Could you check a few things on this model? Use its own coordinates, in mm. Face numbers are marked on the shaded views. A direction names the side the tool comes from. Give positions to 0.01 mm unless a question says otherwise; leave off trailing zeros. Loops run counter-clockwise (first coordinate to the right, second up) from the corner with the lowest first, then second, coordinate; pieces in that order, holes last. Notation, with made-up numbers: M 63.25,-35.75 L 121.25,-35.75 A16 ccw 121.25,-13.75 Z; hole C 37.5,70 d1. An arc over 180 degrees is marked long. Answer in a Markdown table with one row per item. Add a question column.
1. I need wall thicknesses on line 1 along X through (y, z) = (-2.5, 13); line 2 along X through (y, z) = (-17.5, 19); line 3 along Z through (x, y) = (-15, -4.5). Which ranges of each line are inside material? Lowest first, please. Write a range as from..to.
2. Which directions (+Z, -Z, +X, -X, +Y, -Y) give clear straight access to the entire face, cutting with the end or side of a thin tool? Please do the marked faces 5 and 6.
3. I'm going to push flat-ended pins straight in: pin 1 Ø3.5 at (y, z) = (-38, 16) entering from +X; pin 2 Ø5 at (y, z) = (-13, 3) entering from +X; pin 3 Ø0.9 at (y, z) = (-38, 8.5) entering from +X. Where does each tip first touch, or does it pass through?
4. If we section it at C-C on z = 7.25: List the corners of the cut face in (x, y) for me.
5. If we section it at A-A on z = 11.25: List the corners of the cut face in (x, y) for me, then the cut area to 3 significant figures.
6. Thinking about a two-plate mould opening in Z: for the marked faces 1, 2, 3 and 4, which applies, released by +Z, released by -Z, zero draft, split by the parting line, or undercut?
7. If we section it at B-B on x = -8: List the corners of the cut face in (y, z) for me.
8. If we section it at D-D on x = 2: List the corners of the cut face in (y, z) for me.
```python
from build123d import *

# Parameters (mm, degrees)
F0_W          = 54.9165850133
F0_H          = 29.332328558
F1_DEPTH      = 25
F2_W          = 54.8067912459
F2_H          = 9.8693305627
F3_DEPTH      = 10
F3_DEPTH_BACK = 25
F4_DEPTH      = 3
F5_R          = 5
F6_W          = 44.9165850133
F6_H          = 6.1664939672
F6_H_2        = 4.8576648161
F7_DEPTH      = 3


with BuildPart() as f1:
    # F0 (on Top) → F1 (new body)
    with BuildSketch(Plane.XY):
        with Locations((-0.0417074934, -24.666164279)):
            Rectangle(F0_W, F0_H)
        Polygon((27.5, 10), (-27.5, 10), (-27.5, -10), (27.4165850133, -10), (27.5, -10), align=None)
        Polygon((-22.7641869603, -1.5628831632), (-22.7355900026, 1.6124145468), (-19.9714030424, 3.17529771), (-17.2358130397, 1.5628831632), (-17.2644099974, -1.6124145468), (-20.0285969576, -3.17529771), align=None, mode=Mode.SUBTRACT)
        Polygon((2.7641869603, 1.5628831632), (2.7355900026, -1.6124145468), (-0.0285969576, -3.17529771), (-2.7641869603, -1.5628831632), (-2.7355900026, 1.6124145468), (0.0285969576, 3.17529771), align=None, mode=Mode.SUBTRACT)
        Polygon((22.7641869603, 1.5628831632), (22.7355900026, -1.6124145468), (19.9714030424, -3.17529771), (17.2358130397, -1.5628831632), (17.2644099974, 1.6124145468), (20.0285969576, 3.17529771), align=None, mode=Mode.SUBTRACT)
    extrude(amount=F1_DEPTH)

    # F2 (on Front) → F3 (cut, two sides)
    with BuildSketch(Plane.XZ) as f3_sk:
        with Locations((-0.1290403306, 4.9346652813)):
            Rectangle(F2_W, F2_H)
    extrude(amount=F3_DEPTH, mode=Mode.SUBTRACT)
    extrude(f3_sk.sketch, amount=-F3_DEPTH_BACK, mode=Mode.SUBTRACT)

    # F0 (on Top) → F4 (join)
    with BuildSketch(Plane.XY):
        Polygon((27.5, 10), (-27.5, 10), (-27.5, -10), (27.4165850133, -10), (27.5, -10), align=None)
        Polygon((-22.7641869603, -1.5628831632), (-22.7355900026, 1.6124145468), (-19.9714030424, 3.17529771), (-17.2358130397, 1.5628831632), (-17.2644099974, -1.6124145468), (-20.0285969576, -3.17529771), align=None, mode=Mode.SUBTRACT)
        Polygon((2.7641869603, 1.5628831632), (2.7355900026, -1.6124145468), (-0.0285969576, -3.17529771), (-2.7641869603, -1.5628831632), (-2.7355900026, 1.6124145468), (0.0285969576, 3.17529771), align=None, mode=Mode.SUBTRACT)
        Polygon((22.7641869603, 1.5628831632), (22.7355900026, -1.6124145468), (19.9714030424, -3.17529771), (17.2358130397, -1.5628831632), (17.2644099974, 1.6124145468), (20.0285969576, 3.17529771), align=None, mode=Mode.SUBTRACT)
    extrude(amount=F4_DEPTH)

    # F5
    f5_edges = [f1.edges().sort_by_distance(p)[0] for p in [
        (-0.041707, -39.332329, 25),
        (-0.041707, -39.332329, 0),
        (27.416585, -39.332329, 12.5),
        (-27.5, -39.332329, 12.5),
    ]]
    fillet(f5_edges, radius=F5_R)

    # F6 (on face) → F7 (cut)
    with BuildSketch(Plane.XZ.offset(39.332328558)):
        with Locations((-0.0417074934, 16.9167530164)):
            Rectangle(F6_W, F6_H)
        with Locations((-0.0417074934, 7.428832408)):
            Rectangle(F6_W, F6_H_2)
    extrude(amount=-F7_DEPTH, mode=Mode.SUBTRACT)


solid = f1.part
```
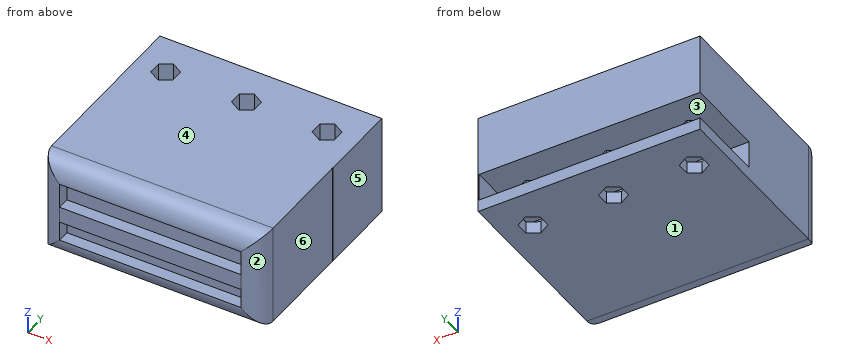
Results:
| question | item | result |
|---|---|---|
| 1 | line 1 | -27.5..-21.17, -18.83..-1.17, 1.17..18.83, 21.17..27.5 |
| 1 | line 2 | -27.5..27.42 |
| 1 | line 3 | 0..3, 9.87..25 |
| 2 | face 5 | +Z, -Z, +X, +Y, -Y |
| 2 | face 6 | +Z, -Z, +X, -Y |
| 3 | pin 1 | x = 27.03 |
| 3 | pin 2 | x = 27.42 |
| 3 | pin 3 | x = 26.24 |
| 4 | outline | M -27.5,-34.33 A5 ccw -22.5,-39.33 L -22.5,-36.33 L 22.42,-36.33 L 22.42,-39.33 A5 ccw 27.42,-34.33 L 27.42,-10 L 27.5,-10 L 27.5,10 L 27.27,10 L 27.27,-10 L -27.5,-10 Z |
| 5 | outline | M -27.5,-34.33 A5 ccw -22.5,-39.33 L 22.42,-39.33 A5 ccw 27.42,-34.33 L 27.42,-10 L 27.5,-10 L 27.5,10 L -27.5,10 Z; hole M -22.76,-1.56 L -20.03,-3.18 L -17.26,-1.61 L -17.24,1.56 L -19.97,3.18 L -22.74,1.61 Z; hole M -2.76,-1.56 L -0.03,-3.18 L 2.74,-1.61 L 2.76,1.56 L 0.03,3.18 L -2.74,1.61 Z; hole M 17.24,-1.56 L 19.97,-3.18 L 22.74,-1.61 L 22.76,1.56 L 20.03,3.18 L 17.26,1.61 Z |
| 5 | area | 2,620 mm2 |
| 6 | face 1 | released by -Z |
| 6 | face 2 | zero draft |
| 6 | face 3 | undercut |
| 6 | face 4 | released by +Z |
| 7 | outline | M -39.33,5 A5 ccw -34.33,0 L 10,0 L 10,3 L -10,3 L -10,9.87 L 10,9.87 L 10,25 L -34.33,25 A5 ccw -39.33,20 L -36.33,20 L -36.33,13.83 L -39.33,13.83 L -39.33,9.86 L -36.33,9.86 L -36.33,5 Z |
| 8 | outline | M -39.33,5 A5 ccw -34.33,0 L -2.03,0 L -2.03,3 L -10,3 L -10,9.87 L -2.03,9.87 L -2.03,25 L -34.33,25 A5 ccw -39.33,20 L -36.33,20 L -36.33,13.83 L -39.33,13.83 L -39.33,9.86 L -36.33,9.86 L -36.33,5 Z; M 2.01,0 L 10,0 L 10,3 L 2.01,3 Z; M 2.01,9.87 L 10,9.87 L 10,25 L 2.01,25 Z |
